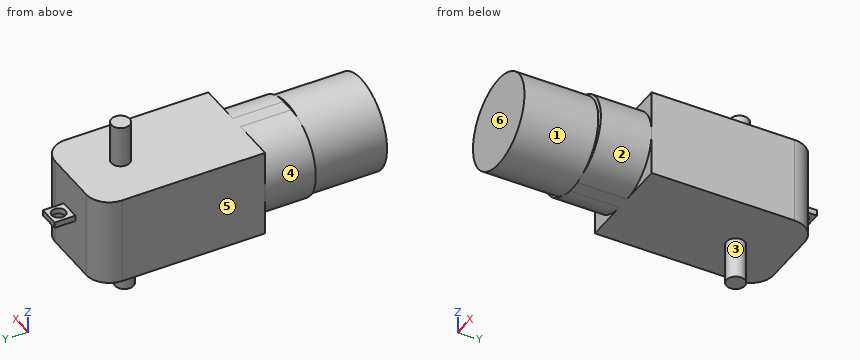
from build123d import *

# Parameters (mm, degrees)
SKETCH_1_W          = 22
SKETCH_1_H          = 36
EXTRUDE_1_DEPTH     = 19
SKETCH_2_W          = 4.5
SKETCH_2_H          = 4.5
EXTRUDE_2_DEPTH     = 1.25
SKETCH_3_R          = 1.5
CUT_EXTRUDE_1_DEPTH = 48.442728631
EXTRUDE_3_DEPTH     = 11
SKETCH_5_R          = 10
EXTRUDE_4_DEPTH     = 16
FILLET_1_R          = 5
SKETCH_6_R          = 2
EXTRUDE_5_DEPTH     = 9
SKETCH_7_R          = 2
EXTRUDE_6_DEPTH     = 9


with BuildPart() as part:
    # ｽｹｯﾁ1 → ﾎﾞｽ - 押し出し1 (new body)
    with BuildSketch(Plane.XY):
        with Locations((11, 18)):
            Rectangle(SKETCH_1_W, SKETCH_1_H)
    extrude(amount=EXTRUDE_1_DEPTH)

    # ｽｹｯﾁ2 → ﾎﾞｽ - 押し出し2 (add)
    with BuildSketch(Plane.XY.offset(10)):
        with Locations((11.44003241, 38.25)):
            Rectangle(SKETCH_2_W, SKETCH_2_H)
    extrude(amount=EXTRUDE_2_DEPTH)

    # ｽｹｯﾁ3 → ｶｯﾄ - 押し出し1 (cut, through all)
    with BuildSketch(Plane.XY.offset(11.25)):
        with Locations((11.478404316, 38.342178873)):
            Circle(SKETCH_3_R)
    extrude(amount=-CUT_EXTRUDE_1_DEPTH, mode=Mode.SUBTRACT)

    # ｽｹｯﾁ4 → ﾎﾞｽ - 押し出し3 (add)
    with BuildSketch(Plane.XZ):
        with BuildLine():
            Line((9.5, 19), (12.5, 19))
            ThreePointArc((12.5, 19), (22, 9.5), (12.5, 0))
            Line((12.5, 0), (9.5, 0))
            ThreePointArc((9.5, 0), (0, 9.5), (9.5, 19))
        make_face()
    extrude(amount=EXTRUDE_3_DEPTH)

    # ｽｹｯﾁ5 → ﾎﾞｽ - 押し出し4 (add)
    with BuildSketch(Plane.XZ.offset(11)):
        with Locations(Location((11, 9.5, 0), (0, 0, 113.578178478))):
            Circle(SKETCH_5_R)
    extrude(amount=EXTRUDE_4_DEPTH)

    # ﾌｨﾚｯﾄ1
    fillet_1_edges = [part.edges().sort_by_distance(p)[0] for p in [
        (0, 36, 9.5),
        (22, 36, 9.5),
    ]]
    fillet(fillet_1_edges, radius=FILLET_1_R)

    # ｽｹｯﾁ6 → ﾎﾞｽ - 押し出し5 (add)
    with BuildSketch(Plane(origin=(0, 0, 0), x_dir=(-1, 0, 0), z_dir=(0, 0, -1))):
        with Locations((-9.86884227, 25)):
            Circle(SKETCH_6_R)
    extrude(amount=EXTRUDE_5_DEPTH)

    # ｽｹｯﾁ7 → ﾎﾞｽ - 押し出し6 (add)
    with BuildSketch(Plane.XY.offset(19)):
        with Locations(Location((11.335077521, 25, 0), (0, 0, 180))):
            Circle(SKETCH_7_R)
    extrude(amount=EXTRUDE_6_DEPTH)


solid = part.part
Build history of the part. All positions in model axes, mm. Face numbers are marked on the shaded views. A direction names the side the tool comes from. Coordinates: 2 decimals unless noted, no trailing zeros. Write each loop counter-clockwise with the first axis right and the second up, starting at its lowest first coordinate (ties: lowest second). Pieces come first, ordered by that corner, then holes.
(1) Cut at A-A on x = 11. List the corners of the cut face in (y, z), and give its area (3 significant figures).
(2) Cut at D-D on z = -3. List the corners of the cut face in (x, y).
(3) Drill centre lines: line 1 (Z direction, x = 5.5, y = 16); line 2 (Y direction, x = 13.5, z = 13); line 3 (Y direction, x = 10, z = -5). Where is each one in solid material? Low to high.
(4) Pin check, flat tips, straight feed: pin 1 Ø1 at (y, z) = (15, 20.5) entering from +X; pin 2 Ø5 at (y, z) = (-20, 16) entering from +X; pin 3 Ø2 at (x, y) = (18, 11.5) entering from +Z; pin 4 Ø1 at (y, z) = (38.5, 10.5) entering from -X. Stop position of each tip, or through.
(5) Cut at C-C on z = 14. List the corners of the cut face in (x, y).
(6) 3-axis set-ups, long thin cutter, end or side, ignore diameter. For the marked faces 1, 2 and 3: which of +Z, -Z, +X, -X, +Y, -Y reach the whole face in a straight line?
(7) Cut at B-B on y = 25. List the corners of the cut face in (x, z).
(8) Mould opens along Y. For the marked faces 4, 5 and 6 say: pulls with the +Y half, pulls with the -Y half, needs draft (parallel to the pull), parting line crosses it, or undercut.
Working result:
1. outline: (-27, -0.5) - (-11, -0.5) - (-11, 0) - (23.35, 0) - (23.35, -9) - (26.65, -9) - (26.65, 0) - (36, 0) - (36, 10) - (36.92, 10) - (36.92, 11.25) - (36, 11.25) - (36, 19) - (26.97, 19) - (26.97, 28) - (23.03, 28) - (23.03, 19) - (-11, 19) - (-11, 19.5) - (-27, 19.5) - close; (39.76, 10) - (40.5, 10) - (40.5, 11.25) - (39.76, 11.25) - close
1. area: 1,280 mm2
2. outline: circle Ø4 at (9.87, 25)
3. line 1: z = 0 to 19
3. line 2: y = -27 to 36
3. line 3: y = 23 to 27
4. pin 1: passes through
4. pin 2: stops at x = 20.17
4. pin 3: stops at z = 19
4. pin 4: stops at x = 9.19
5. outline: (0, 0) - (1.13, 0) - (1.13, -11) - (2.07, -11) - (2.07, -27) - (19.93, -27) - (19.93, -11) - (20.87, -11) - (20.87, 0) - (22, 0) - (22, 31) arc R5 ccw to (17, 36) - (5, 36) arc R5 ccw to (0, 31) - close
6. face 1: -Y
6. face 2: +X
6. face 3: -Z
7. outline: (0, 0) - (7.87, 0) - (7.87, -9) - (11.87, -9) - (11.87, 0) - (22, 0) - (22, 19) - (13.34, 19) - (13.34, 28) - (9.34, 28) - (9.34, 19) - (0, 19) - close
8. face 4: undercut
8. face 5: needs draft
8. face 6: pulls with the -Y half
